Autodesk Fusion 360 part; units mm, degrees
sketch "Sketch1" plane through (0, 0, 0) normal (0, 0, 1) x (1, 0, 0)
  line L0 (0, 0) -> (20, 0)
  line L1 (20, 0) -> (20, 3.5)
  line L2 (20, 3.5) -> (0, 3.5)
  line L3 (0, 3.5) -> (0, 0)
  line L4 (0, 0) -> (4, 0)
  line L5 (4, 0) -> (4, -4)
  line L6 (4, -4) -> (0, -4)
  line L7 (0, -4) -> (0, 0)
  line L8 (20, 3.5) -> (16, 3.5)
  line L9 (16, 3.5) -> (16, 7.5)
  line L10 (16, 7.5) -> (20, 7.5)
  line L11 (20, 7.5) -> (20, 3.5)
  dimension "d1" = 3.5
  dimension "d2" = 20
  dimension "d3" = 4
  dimension "d4" = 4
  dimension "d5" = 4
  dimension "d6" = 4
extrude "Extrude1" add sketch "Sketch1" along normal blind 34 makes body 1
sketch "Sketch2" plane through (0, 0, 0) normal (0, -1, 0) x (1, 0, 0)
  line L0 (4, 0) -> (20, 0)
  line L1 (20, 0) -> (20, 34)
  line L2 (20, 34) -> (4, 34)
  line L3 (4, 34) -> (4, 0)
  circle A0 centre (10, 27.8) radius 1.75
  circle A1 centre (10, 14.6) radius 1.75
  line L4 (16, 34) -> (4, 34) construction
  point P0 (16, 34)
  point P1 (10, 34)
  dimension "d9" = 3.5
  dimension "d10" = 6.2
  dimension "d11" = 13.2
  dimension "d12" = 3.5
extrude "Extrude2" cut sketch "Sketch2" against normal blind 15 contours A0 | A1 bodies 1
pattern_linear "R-Pattern1" count 3 spacing 80 along (0, 1, 0) of bodies 1 makes body 2 at (8.5369, 83.5, 4.298) makes body 3 at (8.5369, 163.5, 4.298)
sketch "Sketch3" plane through (0, 0, 0) normal (0, 0, 1) x (1, 0, 0)
  line L0 (12, 43.5) -> (32, 43.5)
  line L1 (32, 43.5) -> (32, 40)
  line L2 (32, 40) -> (12, 40)
  line L3 (12, 40) -> (12, 43.5)
  line L4 (12, 40) -> (16, 40)
  line L5 (16, 40) -> (16, 36)
  line L6 (16, 36) -> (12, 36)
  line L7 (12, 36) -> (12, 40)
  line L8 (32, 43.5) -> (28, 43.5)
  line L9 (28, 43.5) -> (28, 47.5)
  line L10 (28, 47.5) -> (32, 47.5)
  line L11 (32, 47.5) -> (32, 43.5)
  line L12 (0, 3.5) -> (0, -4)
  line L13 (4, 0) -> (20, 0)
  dimension "d19" = 20
  dimension "d20" = 3.5
  dimension "d21" = 4
  dimension "d22" = 4
  dimension "d23" = 4
  dimension "d24" = 4
  dimension "d25" = 12
  dimension "d26" = 40
extrude "Extrude3" add sketch "Sketch3" along normal blind 34 separate body makes body 4
sketch "Sketch4" plane through (0, 40, 0) normal (0, -1, 0) x (1, 0, 0)
  line L0 (16, 0) -> (32, 0)
  line L1 (32, 0) -> (32, 34)
  line L2 (32, 34) -> (16, 34)
  line L3 (16, 34) -> (16, 0)
  circle A0 centre (22, 27.8) radius 1.75
  circle A1 centre (22, 14.6) radius 1.75
  line L4 (28, 34) -> (16, 34)
  point P0 (28, 34)
  point P1 (22, 34)
  dimension "d29" = 3.5
  dimension "d30" = 3.5
  dimension "d31" = 6.2
  dimension "d32" = 13.2
extrude "Extrude4" cut sketch "Sketch4" against normal blind 5 contours A0 | A1 bodies 4
pattern_linear "R-Pattern2" count 3 spacing 80 along (0, 1, 0) of bodies 4 makes body 5 at (20.5369, 123.5, 4.298) makes body 6 at (20.5369, 203.5, 4.298)
sketch "Sketch5" plane through (0, 0, 0) normal (0, -1, 0) x (1, 0, 0)
  circle A0 centre (10, 27.8) radius 1.75
  circle A1 centre (10, 14.6) radius 1.75
  line L0 (4, 0) -> (20, 0)
  line L1 (20, 0) -> (20, 34)
  line L2 (20, 34) -> (4, 34)
  line L3 (4, 34) -> (4, 0)
  line L4 (0, 0) -> (32, 0)
  line L5 (32, 0) -> (32, -3.5)
  line L6 (32, -3.5) -> (0, -3.5)
  line L7 (0, -3.5) -> (0, 0)
  line L8 (12.2, -3.5) -> (19.8, -3.5)
  line L9 (19.8, -3.5) -> (19.8, -5.5)
  line L10 (19.8, -5.5) -> (12.2, -5.5)
  line L11 (12.2, -5.5) -> (12.2, -3.5)
  point P0 (32, 0)
  point P1 (16, -3.5)
  point P2 (16, -3.5)
  dimension "d39" = 3.5
  dimension "d40" = 7.6
  dimension "d41" = 2
extrude "Extrude5" add sketch "Sketch5" along normal blind -207.5 and the other way up to surface (-4 mm away) contours L0 L4 L5 L6 L7 L8 | L6 L8 L9 L10 L11 bodies 1 2 3 4 5 6
sketch "Sketch6" plane through (0, 0, 0) normal (0, 0, 1) x (1, 0, 0)
  line L0 (32, 200) -> (16, 200)
  line L1 (16, 200) -> (16, 196)
  line L2 (16, 196) -> (12, 196)
  line L3 (12, 196) -> (12, 203.5)
  line L4 (12, 203.5) -> (28, 203.5)
  line L5 (28, 203.5) -> (28, 207.5)
  line L6 (28, 207.5) -> (0, 207.5)
  line L7 (0, 207.5) -> (0, 163.5)
  line L8 (0, 163.5) -> (16, 163.5)
  line L9 (16, 163.5) -> (16, 167.5)
  line L10 (16, 167.5) -> (20, 167.5)
  line L11 (20, 167.5) -> (20, 160)
  line L12 (20, 160) -> (4, 160)
  line L13 (4, 160) -> (4, 156)
  line L14 (4, 156) -> (0, 156)
  line L15 (0, 156) -> (0, 83.5)
  line L16 (0, 83.5) -> (16, 83.5)
  line L17 (16, 83.5) -> (16, 87.5)
  line L18 (16, 87.5) -> (20, 87.5)
  line L19 (20, 87.5) -> (20, 80)
  line L20 (20, 80) -> (4, 80)
  line L21 (4, 80) -> (4, 76)
  line L22 (4, 76) -> (0, 76)
  line L23 (0, 76) -> (0, 3.5)
  line L24 (0, 3.5) -> (16, 3.5)
  line L25 (16, 3.5) -> (16, 7.5)
  line L26 (16, 7.5) -> (20, 7.5)
  line L27 (20, 7.5) -> (20, 0)
  line L28 (20, 0) -> (4, 0)
  line L29 (4, 0) -> (4, -4)
  line L30 (4, -4) -> (32, -4)
  line L31 (32, -4) -> (32, 40)
  line L32 (32, 40) -> (16, 40)
  line L33 (16, 40) -> (16, 36)
  line L34 (16, 36) -> (12, 36)
  line L35 (12, 36) -> (12, 43.5)
  line L36 (12, 43.5) -> (28, 43.5)
  line L37 (28, 43.5) -> (28, 47.5)
  line L38 (28, 47.5) -> (32, 47.5)
  line L39 (32, 47.5) -> (32, 120)
  line L40 (32, 120) -> (16, 120)
  line L41 (16, 120) -> (16, 116)
  line L42 (16, 116) -> (12, 116)
  line L43 (12, 116) -> (12, 123.5)
  line L44 (12, 123.5) -> (28, 123.5)
  line L45 (28, 123.5) -> (28, 127.5)
  line L46 (28, 127.5) -> (32, 127.5)
  line L47 (32, 127.5) -> (32, 200)
  circle A0 centre (16, 182.5) radius 3.2
  line L48 (19.8, 207.5) -> (12.2, 207.5)
  circle A1 centre (16, 101) radius 3.2
  circle A2 centre (16, 19.5) radius 3.2
  point P0 (16, 207.5)
  dimension "d46" = 6.4
  dimension "d47" = 25
  dimension "d50" = 163
  dimension "d51" = 0
extrude "Extrude6" cut sketch "Sketch6" against normal blind 15 contours A0 | A1 | A2 bodies 1
chamfer "Chamfer1" distance 4 angle 45 12 edges at (12, 0, 0) (8, 3.5, 0) (24, 40, 0) (20, 43.5, 0) (12, 80, 0) (8, 83.5, 0) (20, 123.5, 0) (24, 120, 0) (12, 160, 0) (8, 163.5, 0) (24, 200, 0) (20, 203.5, 0) on bodies 1
chamfer "Chamfer2" distance 3 angle 45 6 edges at (12, 201.75, 0) (20, 161.75, 0) (20, 81.75, 0) (20, 1.75, 0) (12, 121.75, 0) (12, 41.75, 0) on bodies 1
chamfer "Chamfer3" distance 1.5 angle 45 12 edges at (32, 200, 19) (12, 203.5, 19) (20, 160, 19) (0, 163.5, 19) (12, 123.5, 19) (32, 120, 19) (20, 80, 19) (0, 83.5, 19) (12, 43.5, 19) (32, 40, 19) (20, 0, 19) (0, 3.5, 19) on bodies 1
equation "d12 = d9"
equation "d22 = d21"
equation "d23 = d21"
equation "d24 = d21"
Input: part model. Units: mm. Frame: model coordinates. A direction names the side the tool comes from. Coordinates: 2 decimals unless noted, no trailing zeros. Loops run counter-clockwise (first coordinate to the right, second up) from the corner with the lowest first, then second, coordinate; pieces in that order, holes last. Notation, with made-up numbers: (82.5, 27.25) - (104.5, 27.25) arc R29 cw to (104.5, 51.25) - close; hole circle Ø1 at (71.25, -21.5). An arc over 180 degrees is marked (long way). Answer in a Markdown table with one row per item. Add a question column.
Item 1: Section query A-A on y = 101. Return the cut outline in (x, z).
Item 2: Mould query, pull axis Y, two halves, no side actions, for faces 1 (the cylindrical face through (20.25, 201.73, 14.68)), 2 (the flat face through (18, 87.5, 17)), 3 (the flat face through (18.6, 205.3, 2.2)). Classes: released by +Y, released by -Y, zero draft, split by the parting line, or undercut.
Item 3: Access query for faces 4 (the flat face through (21, 203.5, 19)), 5 (the flat face through (6, 100, -3.5)), 6 (the flat face through (20, 84, 18)), 7 (the flat face through (21, 43.5, 19)). Directions: +Z, -Z, +X, -X, +Y, -Y. A direction counts if a zero-diameter tool reaches every point of the face in a straight line with its end or side. Return the directions, or none.
Item 4: Contact query for flat-ended pins moving along their axis: P1, Ø6, axis at x = 25.5, y = 100.5, coming from the -Z side; P2, Ø9.5, axis at y = 4, z = 13, coming from the +X side; P3, Ø8.5, axis at x = 16, y = 182.5, coming from the +Z side. Output: stop coordinate, or through.
Item 5: Section query D-D on z = 22. State how many separate pieces and enclosed holes the cut face has, then the cut area to 4 significant figures.
Item 6: Section query B-B on y = 70.5. Return the cut outline in (x, z), then the cut area to 3 significant figures.
Item 7: Line query: line 1 along Y through (x, z) = (15, 29); line 2 along Y through (x, z) = (18.5, 13); line 3 along Y through (x, z) = (16, -3). Output: solid intervals per line, ascending. Write a range as [from, to].
Recorded:
| question | item | result |
|---|---|---|
| 1 | outline | (0, -3.5) - (12.2, -3.5) - (12.2, -5.5) - (12.8, -5.5) - (12.8, 0) - (0, 0) - close; (19.2, -5.5) - (19.8, -5.5) - (19.8, -3.5) - (32, -3.5) - (32, 0) - (19.2, 0) - close |
| 2 | face 1 | zero draft |
| 2 | face 2 | undercut |
| 2 | face 3 | released by +Y |
| 3 | face 4 | +Z, -X, +Y |
| 3 | face 5 | -Z, -X, +Y, -Y |
| 3 | face 6 | +Z, +X |
| 3 | face 7 | +Z, -X |
| 4 | P1 | z = -3.5 |
| 4 | P2 | x = 20 |
| 4 | P3 | z = 0 |
| 5 | separate pieces | 6 |
| 5 | enclosed holes | 0 |
| 5 | area | 598.5 mm^2 |
| 6 | outline | (0, -3.5) - (12.2, -3.5) - (12.2, -5.5) - (19.8, -5.5) - (19.8, -3.5) - (32, -3.5) - (32, 0) - (0, 0) - close |
| 6 | area | 127 mm^2 |
| 7 | line 1 | [0, 3.5], [36, 43.5], [80, 83.5], [116, 123.5], [160, 163.5], [196, 203.5] |
| 7 | line 2 | [0, 7.5], [40, 43.5], [80, 87.5], [120, 123.5], [160, 167.5], [200, 203.5] |
| 7 | line 3 | [-4, 16.3], [22.7, 97.8], [104.2, 179.3], [185.7, 207.5] |
